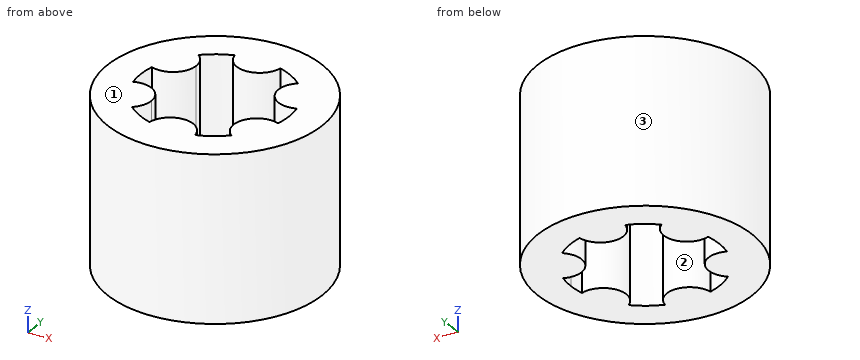
from build123d import *

# Parameters (mm, degrees)
F0_R     = 3.25
F1_DEPTH = 5


with BuildPart() as f1:
    # F0 (on Top) → F1 (new body)
    with BuildSketch(Plane.XY):
        Circle(F0_R)
        with BuildLine():
            ThreePointArc((2.1999961154, 0.4717171738), (2.2374641069, 0.2371800374), (2.25, 0))
            ThreePointArc((2.25, 0), (2.2374641069, -0.2371800374), (2.1999961154, -0.4717171738))
            ThreePointArc((2.1999961154, -0.4717171738), (2.5256218299, -0.7287723318), (2.6485571585, -1.125))
            ThreePointArc((2.6485571585, -1.125), (2.2501959894, -1.7566755621), (1.5085171137, -1.6693939373))
            ThreePointArc((1.5085171137, -1.6693939373), (1.125, -1.9485571585), (0.6914790018, -2.1411111111))
            ThreePointArc((0.6914790018, -2.1411111111), (0.6978664991, -2.1953891093), (0.7, -2.25))
            ThreePointArc((0.7, -2.25), (-0.0546108907, -2.9478664991), (-0.6914790018, -2.1411111111))
            ThreePointArc((-0.6914790018, -2.1411111111), (-1.125, -1.9485571585), (-1.5085171137, -1.6693939373))
            ThreePointArc((-1.5085171137, -1.6693939373), (-2.5547749412, -1.475), (-2.1999961154, -0.4717171738))
            ThreePointArc((-2.1999961154, -0.4717171738), (-2.25, 0), (-2.1999961154, 0.4717171738))
            ThreePointArc((-2.1999961154, 0.4717171738), (-2.5547749412, 1.475), (-1.5085171137, 1.6693939373))
            ThreePointArc((-1.5085171137, 1.6693939373), (-1.125, 1.9485571585), (-0.6914790018, 2.1411111111))
            ThreePointArc((-0.6914790018, 2.1411111111), (-0.0546108907, 2.9478664991), (0.7, 2.25))
            ThreePointArc((0.7, 2.25), (0.6978664991, 2.1953891093), (0.6914790018, 2.1411111111))
            ThreePointArc((0.6914790018, 2.1411111111), (1.125, 1.9485571585), (1.5085171137, 1.6693939373))
            ThreePointArc((1.5085171137, 1.6693939373), (2.2501959894, 1.7566755621), (2.6485571585, 1.125))
            ThreePointArc((2.6485571585, 1.125), (2.5256218299, 0.7287723318), (2.1999961154, 0.4717171738))
        make_face(mode=Mode.SUBTRACT)
        with BuildLine():
            ThreePointArc((1.5085171137, 1.6693939373), (1.9485571585, 1.125), (2.1999961154, 0.4717171738))
            ThreePointArc((2.1999961154, 0.4717171738), (2.5256218299, 0.7287723318), (2.6485571585, 1.125))
            ThreePointArc((2.6485571585, 1.125), (2.2501959894, 1.7566755621), (1.5085171137, 1.6693939373))
        make_face()
        with BuildLine():
            ThreePointArc((2.6485571585, -1.125), (2.5256218299, -0.7287723318), (2.1999961154, -0.4717171738))
            ThreePointArc((2.1999961154, -0.4717171738), (1.9485571585, -1.125), (1.5085171137, -1.6693939373))
            ThreePointArc((1.5085171137, -1.6693939373), (2.2501959894, -1.7566755621), (2.6485571585, -1.125))
        make_face()
        with BuildLine():
            ThreePointArc((-0.6914790018, 2.1411111111), (0, 2.25), (0.6914790018, 2.1411111111))
            ThreePointArc((0.6914790018, 2.1411111111), (0.6978664991, 2.1953891093), (0.7, 2.25))
            ThreePointArc((0.7, 2.25), (-0.0546108907, 2.9478664991), (-0.6914790018, 2.1411111111))
        make_face()
        with BuildLine():
            ThreePointArc((0.7, -2.25), (0.6978664991, -2.1953891093), (0.6914790018, -2.1411111111))
            ThreePointArc((0.6914790018, -2.1411111111), (0, -2.25), (-0.6914790018, -2.1411111111))
            ThreePointArc((-0.6914790018, -2.1411111111), (-0.0546108907, -2.9478664991), (0.7, -2.25))
        make_face()
        with BuildLine():
            ThreePointArc((-2.1999961154, 0.4717171738), (-1.9485571585, 1.125), (-1.5085171137, 1.6693939373))
            ThreePointArc((-1.5085171137, 1.6693939373), (-2.5547749412, 1.475), (-2.1999961154, 0.4717171738))
        make_face()
        with BuildLine():
            ThreePointArc((-2.1999961154, -0.4717171738), (-2.5547749412, -1.475), (-1.5085171137, -1.6693939373))
            ThreePointArc((-1.5085171137, -1.6693939373), (-1.9485571585, -1.125), (-2.1999961154, -0.4717171738))
        make_face()
        with BuildLine():
            ThreePointArc((1.5085171137, 1.6693939373), (1.3423393759, 0.775), (2.1999961154, 0.4717171738))
            ThreePointArc((2.1999961154, 0.4717171738), (1.9485571585, 1.125), (1.5085171137, 1.6693939373))
        make_face()
        with BuildLine():
            ThreePointArc((1.5085171137, -1.6693939373), (1.9485571585, -1.125), (2.1999961154, -0.4717171738))
            ThreePointArc((2.1999961154, -0.4717171738), (1.3423393759, -0.775), (1.5085171137, -1.6693939373))
        make_face()
        with BuildLine():
            ThreePointArc((-0.6914790018, 2.1411111111), (0, 1.55), (0.6914790018, 2.1411111111))
            ThreePointArc((0.6914790018, 2.1411111111), (0, 2.25), (-0.6914790018, 2.1411111111))
        make_face()
        with BuildLine():
            ThreePointArc((-0.6914790018, -2.1411111111), (0, -2.25), (0.6914790018, -2.1411111111))
            ThreePointArc((0.6914790018, -2.1411111111), (0, -1.55), (-0.6914790018, -2.1411111111))
        make_face()
        with BuildLine():
            ThreePointArc((-1.2485571585, 1.125), (-1.3168815965, 1.4266388309), (-1.5085171137, 1.6693939373))
            ThreePointArc((-1.5085171137, 1.6693939373), (-1.9485571585, 1.125), (-2.1999961154, 0.4717171738))
            ThreePointArc((-2.1999961154, 0.4717171738), (-1.5523294903, 0.5479353287), (-1.2485571585, 1.125))
        make_face()
        with BuildLine():
            ThreePointArc((-2.1999961154, -0.4717171738), (-1.9485571585, -1.125), (-1.5085171137, -1.6693939373))
            ThreePointArc((-1.5085171137, -1.6693939373), (-1.3168815965, -1.4266388309), (-1.2485571585, -1.125))
            ThreePointArc((-1.2485571585, -1.125), (-1.5523294903, -0.5479353287), (-2.1999961154, -0.4717171738))
        make_face()
    extrude(amount=F1_DEPTH)


solid = f1.part
The model under review builds one solid part; all positions refer to its coordinate system, in mm. Face numbers are marked on the shaded views. Round coordinates to 2 decimals unless told otherwise and drop trailing zeros. Write each loop counter-clockwise with the first axis right and the second up, starting at its lowest first coordinate (ties: lowest second). Pieces come first, ordered by that corner, then holes. Notation, with made-up numbers: (66.5, 65) - (89.5, 65) arc R29 cw to (89.5, 90) - close; hole circle Ø7 at (54.5, 31.25). An arc over 180 degrees is marked (long way). One line per item, written item: value. Start each with the question number.
1. The part is to be moulded in two halves that separate along X. For the marked faces 1, 2 and 3, say which applies: released by +X, released by -X, zero draft, split by the parting line, or undercut.
2. Clearance check with flat-ended pins moving along their axes: P1, Ø1.5, axis at y = 2, z = 2.5, coming from the +X side; P2, Ø1, axis at x = 1, z = 2.5, coming from the -Y side; P3, Ø2, axis at y = 2, z = 0.5, coming from the -X side. State where each tip first meets the part, or that it passes through.
3. Consider section A-A on x = 0. Write out the cut boundary in (y, z).
4. Consider section C-C on z = 1.4. Write out the cut boundary in (x, y) (3 decimals), and give its area (3 significant figures).
5. To check wall thickness, follow L1, parallel to X at y = -1.75, z = 0.25; L2, parallel to X at y = 0.75, z = 0.55; L3, parallel to Y at x = 0, z = 1.25. State the ranges of each line that lie inside material, in increasing order. Write a range as from..to.
6. Consider section B-B on y = 1. Write out the cut boundary in (x, z).
7. Consider section D-D on x = 2.5. Write out the cut boundary in (y, z).
Checks:
1. face 1: zero draft
1. face 2: undercut
1. face 3: split by the parting line
2. P1: stops at x = 3
2. P2: stops at y = -3.21
2. P3: stops at x = -3.09
3. outline: (-3.25, 0) - (-1.55, 0) - (-1.55, 5) - (-3.25, 5) - close; (1.55, 0) - (3.25, 0) - (3.25, 5) - (1.55, 5) - close
4. outline: circle Ø6.5 at (0, 0); hole (-2.2, -0.472) arc R0.7 cw to (-1.509, -1.669) arc R2.25 ccw to (-0.691, -2.141) arc R0.7 cw to (0.691, -2.141) arc R2.25 ccw to (1.509, -1.669) arc R0.7 cw to (2.2, -0.472) arc R2.25 ccw to (2.2, 0.472) arc R0.7 cw to (1.509, 1.669) arc R2.25 ccw to (0.691, 2.141) arc R0.7 cw to (-0.691, 2.141) arc R2.25 ccw to (-1.509, 1.669) arc R0.7 cw to (-2.2, 0.472) arc R2.25 ccw to start
4. area: 21.6 mm^2
5. L1: x = -2.74..-1.41, -0.49..0.49, 1.41..2.74
5. L2: x = -3.16..-1.36, 1.36..3.16
5. L3: y = -3.25..-1.55, 1.55..3.25
6. outline: (-3.09, 0) - (-1.26, 0) - (-1.26, 5) - (-3.09, 5) - close; (1.26, 0) - (3.09, 0) - (3.09, 5) - (1.26, 5) - close
7. outline: (-2.08, 0) - (2.08, 0) - (2.08, 5) - (-2.08, 5) - close
